from build123d import *

# Parameters (mm, degrees)
F1_DEPTH = 6
F2_R     = 1.5
F2_R_2   = 1.85
F3_DEPTH = 25


with BuildPart() as f1:
    # F0 (on Top) → F1 (new body)
    with BuildSketch(Plane.XY):
        with BuildLine():
            Line((-18.5, -9), (18.5, -9))
            Line((18.5, -9), (18.5, 9))
            Line((18.5, 9), (1.5, 9))
            Line((1.5, 9), (-3.5, 9))
            ThreePointArc((-3.5, 9), (-7.035534, 10.464466), (-8.5, 14))
            Line((-8.5, 14), (-8.5, 81))
            Line((-8.5, 81), (-18.5, 81))
            Line((-18.5, 81), (-23.5, 81))
            Line((-23.5, 81), (-23.5, 76))
            Line((-23.5, 76), (-18.5, 76))
            Line((-18.5, 76), (-18.5, 9))
            Line((-18.5, 9), (-18.5, -9))
        make_face()
    extrude(amount=F1_DEPTH)

    # F2 (on face) → F3 (cut)
    with BuildSketch(Plane.XY.offset(6)):
        with Locations((-13.5, -0.5)):
            Circle(F2_R)
        with Locations((13.2, 0)):
            Circle(F2_R_2)
    extrude(amount=-F3_DEPTH, mode=Mode.SUBTRACT)


solid = f1.part
Input: part model. Units: mm. Frame: model coordinates. A direction names the side the tool comes from. Give positions to 0.01 mm unless a question says otherwise; leave off trailing zeros. Write each loop counter-clockwise with the first axis right and the second up, starting at its lowest first coordinate (ties: lowest second). Pieces come first, ordered by that corner, then holes. Notation, with made-up numbers: (-13, 65.25) -> (41, 65.25) arc R21 ccw to (41, 74.25) -> close; hole circle Ø7 at (-15.75, 33). An arc over 180 degrees is marked (long way). Use one line per item in the form item = value. Start each with the question number.
1) Section query B-B on z = 3.6. Return the cut outline in (x, y), then the cut area to 3 significant figures.
2) Section query C-C on x = -13.5. Return the cut outline in (y, z), then the cut area to 3 significant figures.
3) Set-up query: faces 1 (the flat face through (-8.5, 47, 3)), 2 (the flat face through (-18.5, 34, 3)), 3 (the flat face through (18.5, 0, 3)). Return all of +Z, -Z, +X, -X, +Y, -Y with unobstructed straight access to the full face (end or side cutting, diameter ignored); none if empty.
4) Section query A-A on x = 13.2. Return the cut outline in (y, z).
5) Pin query (flat end, axial travel): pin 1 (1.8 mm diameter, centred on x = 11, z = 3.5, fed in from +Y); pin 2 (1.5 mm diameter, centred on y = 32, z = 3, fed in from -X); pin 3 (1.5 mm diameter, centred on y = 45, z = 5.5, fed in from +X). Return the tip coordinate at first contact, or that it passes through.
6) Ray query, probe 1 along Y at (x, z) = (-13.5, 4.05); probe 2 along Y at (x, z) = (13.2, 3.25); probe 3 along X at (y, z) = (33, 2.8). Return the intervals inside material, ascending. Write a range as from..to.
7) Draft query along X for faces 4 (the cylindrical face through (-15, -0.43, 3.04)), 5 (the cylindrical face through (14.91, -0.71, 3.04)), 6 (the flat face through (8, 9, 3)), 7 (the flat face through (-23.5, 79, 3)). Return one class per face: pulls with the +X half, pulls with the -X half, needs draft (parallel to the pull), parting line crosses it, or undercut.
8) Section query D-D on y = 49.5. Return the cut outline in (x, z).
Outcome:
q1.outline = (-23.5, 76) -> (-18.5, 76) -> (-18.5, -9) -> (18.5, -9) -> (18.5, 9) -> (-3.5, 9) arc R5 cw to (-8.5, 14) -> (-8.5, 81) -> (-23.5, 81) -> close; hole circle Ø3 at (-13.5, -0.5); hole circle Ø3.7 at (13.2, 0)
q1.area = 1,400 mm^2
q2.outline = (-9, 0) -> (-2, 0) -> (-2, 6) -> (-9, 6) -> close; (1, 0) -> (81, 0) -> (81, 6) -> (1, 6) -> close
q2.area = 522 mm^2
q3.face_1 = +Z, -Z, +X, +Y
q3.face_2 = +Z, -Z, -X, -Y
q3.face_3 = +Z, -Z, +X, +Y, -Y
q4.outline = (-9, 0) -> (-1.85, 0) -> (-1.85, 6) -> (-9, 6) -> close; (1.85, 0) -> (9, 0) -> (9, 6) -> (1.85, 6) -> close
q5.pin_1 = 9
q5.pin_2 = -18.5
q5.pin_3 = -8.5
q6.probe_1 = -9..-2, 1..81
q6.probe_2 = -9..-1.85, 1.85..9
q6.probe_3 = -18.5..-8.5
q7.face_4 = undercut
q7.face_5 = undercut
q7.face_6 = needs draft
q7.face_7 = pulls with the -X half
q8.outline = (-18.5, 0) -> (-8.5, 0) -> (-8.5, 6) -> (-18.5, 6) -> close
